Check sheet for the modelled part. Datum: model origin and axes. Units: mm. Face numbers are marked on the shaded views. A direction names the side the tool comes from. Give positions to 0.01 mm unless a question says otherwise; leave off trailing zeros. Write each loop counter-clockwise with the first axis right and the second up, starting at its lowest first coordinate (ties: lowest second). Pieces come first, ordered by that corner, then holes. Notation, with made-up numbers: M 64,26.25 L 114,26.25 A20 ccw 114,54.25 Z; hole C 6.5,10.25 d4. An arc over 180 degrees is marked long. Write item = value, one per line. Start each with the question number.
1) Sectioned sample at B-B, the plane z = 0. Record the cut outline in (x, y).
2) Set-up check for the marked faces 1, 2 and 3: record each of +Z, -Z, +X, -X, +Y, -Y from which the full face is reachable in a straight line by a thin tool's end or side.
3) Gauge pin test, flat ends, axial feed: pin 1 (5.5 mm diameter, centred on x = 0, z = 0, fed in from -Y); pin 2 (4 mm diameter, centred on y = 19.5, z = 2.5, fed in from -X); pin 3 (11.5 mm diameter, centred on y = 13, z = -4.5, fed in from +X); pin 4 (6 mm diameter, centred on x = -64.5, z = -2, fed in from -Y). Record the tip position at first contact, or that the pin passes through.
4) Sectioned sample at D-D, the plane x = -62. Record the cut outline in (y, z), then the cut area to 3 significant figures.
5) Sectioned sample at C-C, the plane z = -5. Record the cut outline in (x, y).
6) Sectioned sample at A-A, the plane x = 0. Record the cut outline in (y, z).
7) Draft check along X on the marked faces 4, 5, 6 and 7. Enter one of: pulls with the +X half, pulls with the -X half, needs draft (parallel to the pull), parting line crosses it, or undercut.
8) Scan lines: L1, parallel to Z at x = -62, y = 26.55; L2, parallel to Y at x = -22.5, z = 1.25; L3, parallel to Y at x = -55, z = 1.75. Record each from-to range of solid material in increasing order.
from build123d import *

# Parameters (mm, degrees)
SKETCH1_R          = 3
BASE_FLANGE1_DEPTH = 5
EDGE_FLANGE1_DEPTH = 20
EDGE_FLANGE2_DEPTH = 20
SKETCH15_R         = 4
CUT_EXTRUDE1_DEPTH = 5
CUT_EXTRUDE2_DEPTH = 5


# Sheet-metal steps are written as plain solids
with BuildPart() as part:
    # Sketch1 → Base-Flange1 (new body)
    with BuildSketch(Plane(origin=(0, 0, 0), x_dir=(1, 0, 0), z_dir=(0, 1, 0))):
        with BuildLine():
            Line((-35, 10), (7, 10))
            ThreePointArc((7, 10), (9.121320344, 9.121320344), (10, 7))
            Line((10, 7), (10, -7))
            ThreePointArc((10, -7), (9.121320344, -9.121320344), (7, -10))
            Line((7, -10), (-35, -10))
            Line((-35, -10), (-35, 10))
        make_face()
        with Locations(Location((0, 0, 0), (0, 0, 270))):
            Circle(SKETCH1_R, mode=Mode.SUBTRACT)
    extrude(amount=-BASE_FLANGE1_DEPTH)

    # Edge-Flange1 section (across the edge) → Edge-Flange1 (add)
    with BuildSketch(Plane(origin=(-40, 0, -10), x_dir=(1, 0, 0), z_dir=(0, 0, 1))):
        with BuildLine():
            Line((-5, 5), (-5, 19.4))
            Line((-5, 19.4), (0, 19.4))
            Line((0, 19.4), (0, 5))
            ThreePointArc((0, 5), (1.464466094, 1.464466094), (5, 0))
            Line((5, 0), (5, -5))
            ThreePointArc((5, -5), (-2.071067812, -2.071067812), (-5, 5))
        make_face()
    extrude(amount=EDGE_FLANGE1_DEPTH)

    # Edge-Flange2 section (across the edge) → Edge-Flange2 (add)
    with BuildSketch(Plane(origin=(-45, 24.4, 10), x_dir=(0, -1, 0), z_dir=(0, 0, -1))):
        with BuildLine():
            Line((-5, 5), (-5, 30))
            Line((-5, 30), (0, 30))
            Line((0, 30), (0, 5))
            ThreePointArc((0, 5), (1.464466094, 1.464466094), (5, 0))
            Line((5, 0), (5, -5))
            ThreePointArc((5, -5), (-2.071067812, -2.071067812), (-5, 5))
        make_face()
    extrude(amount=EDGE_FLANGE2_DEPTH)

    # Sketch15 → Cut-Extrude1 (cut)
    with BuildSketch(Plane(origin=(0, 29.4, 0), x_dir=(1, 0, 0), z_dir=(0, 1, 0))):
        with Locations(Location((-62, 0, 0), (0, 0, 180))):
            Circle(SKETCH15_R)
    extrude(amount=-CUT_EXTRUDE1_DEPTH, mode=Mode.SUBTRACT)

    # Sketch16 → Cut-Extrude2 (cut)
    with BuildSketch(Plane(origin=(0, 29.4, 0), x_dir=(1, 0, 0), z_dir=(0, 1, 0))):
        with BuildLine():
            Line((-75, 7), (-75, 10))
            Line((-75, 10), (-72, 10))
            ThreePointArc((-72, 10), (-74.121320344, 9.121320344), (-75, 7))
        make_face()
        with BuildLine():
            Line((-75, -7), (-75, -10))
            Line((-75, -10), (-72, -10))
            ThreePointArc((-72, -10), (-74.121320344, -9.121320344), (-75, -7))
        make_face()
    extrude(amount=-CUT_EXTRUDE2_DEPTH, mode=Mode.SUBTRACT)


solid = part.part
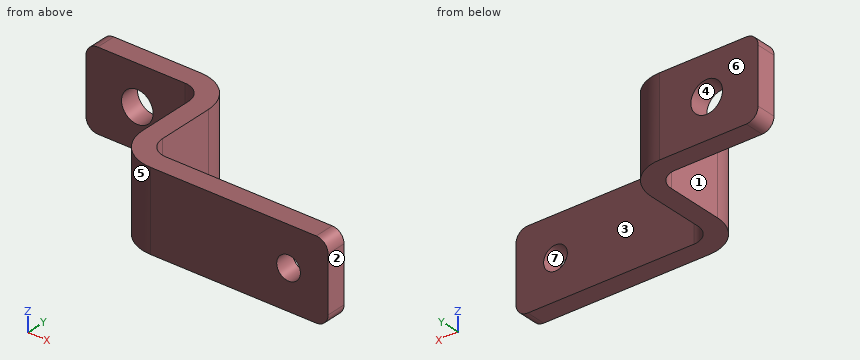
Data:
q1.outline = M -75,24.4 L -66,24.4 L -66,29.4 L -75,29.4 Z; M -58,24.4 L -50,24.4 A5 cw -45,19.4 L -45,5 A10 ccw -35,-5 L -3,-5 L -3,0 L -35,0 A5 cw -40,5 L -40,19.4 A10 ccw -50,29.4 L -58,29.4 Z; M 3,-5 L 10,-5 L 10,0 L 3,0 Z
q2.face_1 = +Z, -Z, -X, -Y
q2.face_2 = +Z, -Z, +X, +Y, -Y
q2.face_3 = +Z, -Z, +X, +Y
q3.pin_1 = through
q3.pin_2 = -45.46
q3.pin_3 = -40
q3.pin_4 = 24.4
q4.outline = M 24.4,-10 L 29.4,-10 L 29.4,-4 L 24.4,-4 Z; M 24.4,4 L 29.4,4 L 29.4,10 L 24.4,10 Z
q4.area = 60.0 mm2
q5.outline = M -75,24.4 L -50,24.4 A5 cw -45,19.4 L -45,5 A10 ccw -35,-5 L 10,-5 L 10,0 L -35,0 A5 cw -40,5 L -40,19.4 A10 ccw -50,29.4 L -75,29.4 Z
q6.outline = M -5,-10 L 0,-10 L 0,-3 L -5,-3 Z; M -5,3 L 0,3 L 0,10 L -5,10 Z
q7.face_4 = undercut
q7.face_5 = pulls with the -X half
q7.face_6 = needs draft
q7.face_7 = undercut
q8.L1 = -10 to -4, 4 to 10
q8.L2 = -5 to 0
q8.L3 = 24.4 to 29.4
